For this review, take the finished solid that the model builds, in its own axes (mm). Face numbers are marked on the shaded views. Give positions to 0.01 mm unless a question says otherwise; leave off trailing zeros. Loops run counter-clockwise (first coordinate to the right, second up) from the corner with the lowest first, then second, coordinate; pieces in that order, holes last.
```python
from build123d import *

# Parameters (mm, degrees)
F0_W     = 32.6
F0_H     = 27
F1_DEPTH = 10
F2_W     = 32.6
F2_H     = 10.75
F3_DEPTH = 0.25
F5_D     = 2.5
F5_DEPTH = 14.2
F5_TIP   = 0.7510757738


with BuildPart() as f1:
    # F0 (on Top) → F1 (new body)
    with BuildSketch(Plane.XY):
        with Locations((16.3, 13.5)):
            Rectangle(F0_W, F0_H)
    extrude(amount=F1_DEPTH)

    # F2 (on face) → F3 (cut)
    with BuildSketch(Plane.XY.offset(10)):
        with Locations((16.3, 13.5)):
            Rectangle(F2_W, F2_H)
    extrude(amount=-F3_DEPTH, mode=Mode.SUBTRACT)

    # F5
    with Locations(Plane.XY.offset(10)):
        with Locations((6.3, 23.5), (26.3, 23.5), (26.3, 3.5), (6.3, 3.5)):
            Hole(F5_D / 2, depth=F5_DEPTH)
            with Locations((0, 0, -(F5_DEPTH + F5_TIP / 2))):  # 118° drill point
                Cone(0, F5_D / 2, F5_TIP, mode=Mode.SUBTRACT)


solid = f1.part
```
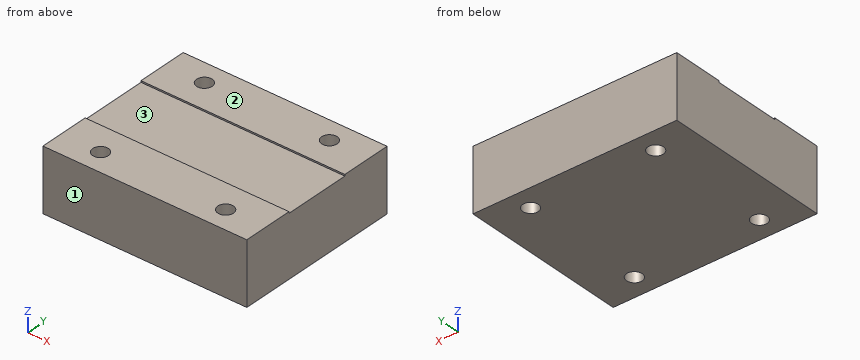
Item 1: Take a section at B-B on x = 26.3. Give the boundary of the cut face in (y, z) (3 decimals).
Answer:
outline: (0, 0) - (2.25, 0) - (2.25, 10) - (0, 10) - close; (4.75, 0) - (22.25, 0) - (22.25, 10) - (18.875, 10) - (18.875, 9.75) - (8.125, 9.75) - (8.125, 10) - (4.75, 10) - close; (24.75, 0) - (27, 0) - (27, 10) - (24.75, 10) - close
Item 2: The part is to be moulded in two halves that separate along Y. For the marked faces 1, 2 and 3, say which applies: released by +Y, released by -Y, zero draft, split by the parting line, or undercut.
Answer:
face 1: released by -Y
face 2: zero draft
face 3: undercut
Item 3: Take a section at D-D on y = 13.5. Give the boundary of the cut face in (x, z).
Answer:
outline: (0, 0) - (32.6, 0) - (32.6, 9.75) - (0, 9.75) - close
Item 4: Take a section at C-C on z = 9. Give the boundary of the cut face in (x, y), and give its area (3 significant figures).
Answer:
outline: (0, 0) - (32.6, 0) - (32.6, 27) - (0, 27) - close; hole circle Ø2.5 at (6.3, 3.5); hole circle Ø2.5 at (6.3, 23.5); hole circle Ø2.5 at (26.3, 3.5); hole circle Ø2.5 at (26.3, 23.5)
area: 861 mm2
Item 5: Take a section at A-A on y = 3.5. Give the boundary of the cut face in (x, z).
Answer:
outline: (0, 0) - (5.05, 0) - (5.05, 10) - (0, 10) - close; (7.55, 0) - (25.05, 0) - (25.05, 10) - (7.55, 10) - close; (27.55, 0) - (32.6, 0) - (32.6, 10) - (27.55, 10) - close
Item 6: For L1, parallel to Y at x = 6.3, z = 4.25; L2, parallel to Z at x = 17, y = 16.25, list the stretches that pass through material, from the lowest coordinate up.
Answer:
L1: y = 0 to 2.25, 4.75 to 22.25, 24.75 to 27
L2: z = 0 to 9.75
Item 7: Clearance check with flat-ended pins moving along their axes: pin 1 Ø1.5 at (x, y) = (6.3, 3.5) entering from +Z; pin 2 Ø3 at (x, y) = (14, 11) entering from +Z. State where each tip first meets the part, or that it passes through.
Answer:
pin 1: passes through
pin 2: stops at z = 9.75
